```python
from build123d import *
from OCP.BRepAlgoAPI import BRepAlgoAPI_Cut
from OCP.TopTools import TopTools_ListOfShape

# Parameters (mm, degrees)
SKETCH1_R                 = 10
SKETCH1_R_2               = 1.35
BOSS_EXTRUDE1_DEPTH       = 3.175
SKETCH2_W                 = 38.058543228
SKETCH2_H                 = 41.75
SKETCH2_R                 = 1.35
BOSS_EXTRUDE2_DEPTH       = 3.175
SKETCH3_W                 = 38.058543228
SKETCH3_H                 = 41.75
SKETCH3_W_2               = 31.708543228
SKETCH3_H_2               = 35.4
BOSS_EXTRUDE3_DEPTH       = 20
FILLET1_R                 = 5
BOSS_EXTRUDE4_OUTLINE_R   = 1
BOSS_EXTRUDE4_OUTLINE_R_2 = 0.698520241
BOSS_EXTRUDE4_OUTLINE_R_3 = 0.699131638
BOSS_EXTRUDE4_DEPTH       = 4.524579022
SKETCH6_R                 = 0.699665004
SKETCH6_R_2               = 0.703272365
SKETCH6_R_3               = 0.700673295
SKETCH6_R_4               = 0.698053945
BOSS_EXTRUDE5_DEPTH       = 5.225420978
CUT_EXTRUDE3_DEPTH        = 39.629021569
CUT_EXTRUDE4_DEPTH        = 44.672508997
FILLET2_R                 = 1


with BuildPart() as part:
    # Sketch1 → Boss-Extrude1 (new body)
    with BuildSketch(Plane(origin=(0, 0, 0), x_dir=(1, 0, 0), z_dir=(0, 1, 0))):
        with Locations(Location((0, 0, 0), (0, 0, 270))):
            Circle(SKETCH1_R)
        with Locations(Location((0, 7, 0), (0, 0, 270))):
            Circle(SKETCH1_R_2, mode=Mode.SUBTRACT)
        with Locations(Location((7, 0, 0), (0, 0, 270))):
            Circle(SKETCH1_R_2, mode=Mode.SUBTRACT)
        with Locations(Location((0, -7, 0), (0, 0, 270))):
            Circle(SKETCH1_R_2, mode=Mode.SUBTRACT)
        with Locations(Location((-7, 0, 0), (0, 0, 270))):
            Circle(SKETCH1_R_2, mode=Mode.SUBTRACT)
    extrude(amount=BOSS_EXTRUDE1_DEPTH)

    # Sketch2 → Boss-Extrude2 (add)
    with BuildSketch(Plane(origin=(0, 3.175, 0), x_dir=(1, 0, 0), z_dir=(0, 1, 0))):
        Rectangle(SKETCH2_W, SKETCH2_H)
        with Locations(Location((0, -7, 0), (0, 0, 270))):
            Circle(SKETCH2_R, mode=Mode.SUBTRACT)
        with Locations(Location((7, 0, 0), (0, 0, 270))):
            Circle(SKETCH2_R, mode=Mode.SUBTRACT)
        with Locations(Location((-7, 0, 0), (0, 0, 270))):
            Circle(SKETCH2_R, mode=Mode.SUBTRACT)
        with Locations(Location((0, 7, 0), (0, 0, 270))):
            Circle(SKETCH2_R, mode=Mode.SUBTRACT)
    extrude(amount=BOSS_EXTRUDE2_DEPTH)

    # Sketch3 → Boss-Extrude3 (add)
    with BuildSketch(Plane(origin=(0, 6.35, 0), x_dir=(1, 0, 0), z_dir=(0, 1, 0))):
        Rectangle(SKETCH3_W, SKETCH3_H)
        Rectangle(SKETCH3_W_2, SKETCH3_H_2, mode=Mode.SUBTRACT)
    extrude(amount=BOSS_EXTRUDE3_DEPTH)

    # Fillet1
    fillet1_edges = [part.edges().sort_by_distance(p)[0] for p in [
        (-19.029271614, 14.7625, -20.875),
        (-19.029271614, 14.7625, 20.875),
        (19.029271614, 14.7625, 20.875),
        (19.029271614, 14.7625, -20.875),
    ]]
    fillet(fillet1_edges, radius=FILLET1_R)

    # Boss-Extrude4: read off the stored shape, not the designer's step
    # Boss-Extrude4 outline → Boss-Extrude4 (add)
    # profile 1 of 2: a face of its own
    with BuildSketch(Plane.XY.offset(16.350420978)):
        with BuildLine():
            ThreePointArc((9.674791631, 35.998523082), (9.427181956, 35.932908065), (9.244559074, 35.753284112))
            ThreePointArc((9.244559074, 35.753284112), (8.147643376, 34.213929311), (6.807481387, 32.880961337))
            Line((6.807481387, 32.880961337), (6.807482447, 6.35))
            Line((6.807482447, 6.35), (11.963760646, 6.35))
            Line((11.963760646, 6.35), (11.963760646, 35.998520144))
            Line((11.963760646, 35.998520144), (9.674791631, 35.998523082))
        make_face()
        with Locations((9.857482447, 33.16)):
            Circle(BOSS_EXTRUDE4_OUTLINE_R, mode=Mode.SUBTRACT)
        with Locations((9.857482447, 12.46)):
            Circle(BOSS_EXTRUDE4_OUTLINE_R, mode=Mode.SUBTRACT)
    # profile 2 of 2: a face of its own
    with BuildSketch(Plane.XY.offset(16.350420978)):
        with BuildLine():
            Line((-12.751066043, 35.998520144), (-12.751066043, 6.35))
            Line((-12.751066043, 6.35), (-7.592517553, 6.35))
            Line((-7.592517553, 6.35), (-7.592516964, 32.880958857))
            ThreePointArc((-7.592516964, 32.880958857), (-8.932679762, 34.213927416), (-10.029597495, 35.753282149))
            ThreePointArc((-10.029597495, 35.753282149), (-10.212218516, 35.932905514), (-10.459826737, 35.998520144))
            Line((-10.459826737, 35.998520144), (-12.751066043, 35.998520144))
        make_face()
        with Locations((-10.642517553, 33.16)):
            Circle(BOSS_EXTRUDE4_OUTLINE_R_2, mode=Mode.SUBTRACT)
        with Locations((-10.642517553, 12.46)):
            Circle(BOSS_EXTRUDE4_OUTLINE_R_3, mode=Mode.SUBTRACT)
    extrude(amount=BOSS_EXTRUDE4_DEPTH)

    # Sketch6 → Boss-Extrude5 (add)
    with BuildSketch(Plane(origin=(0, 0, -15.649579022), x_dir=(-1, 0, 0), z_dir=(0, 0, -1))):
        with BuildLine():
            Line((10.992517553, 24.135), (10.992517553, 30.51))
            Line((10.992517553, 30.51), (7.192517366, 30.510000072))
            Line((7.192517366, 30.510000072), (6.892517553, 30.510000072))
            Line((6.892517553, 30.510000072), (6.892517553, 32.612557612))
            add(Edge.make_bspline(
                [(6.975743415, 32.783855976), (6.958921233, 32.771091761), (6.928542383, 32.73934935), (6.899316538, 32.679660552), (6.892517469, 32.634957243), (6.892517553, 32.612557612)],
                knots=[1.062e-06, 1.062e-06, 1.062e-06, 1.062e-06, 0.322323684, 0.658094096, 1, 1, 1, 1], degree=3, weights=[1, 1, 1, 1, 1, 1]))
            ThreePointArc((6.975743415, 32.783855976), (8.509170356, 34.198162413), (9.744817778, 35.878887355))
            add(Edge.make_bspline(
                [(9.950114528, 35.998516481), (9.923391157, 35.998516414), (9.869066225, 35.989019468), (9.796326784, 35.947026629), (9.759487209, 35.903468994), (9.744817778, 35.878887355)],
                knots=[0, 0, 0, 0, 0.324047023, 0.652881456, 1, 1, 1, 1], degree=3, weights=[1, 1, 1, 1, 1, 1]))
            Line((9.950114528, 35.998516481), (11.752517552, 35.998516481))
            Line((11.752517552, 35.998516481), (13.252517552, 35.998516481))
            Line((13.252517552, 35.998516481), (13.252517552, 6.318190736))
            Line((13.252517552, 6.318190736), (-12.46748245, 6.318190736))
            Line((-12.46748245, 6.318190736), (-12.46748245, 35.998516481))
            Line((-12.46748245, 35.998516481), (-10.96748245, 35.998516481))
            Line((-10.96748245, 35.998516481), (-9.165078771, 35.998516481))
            add(Edge.make_bspline(
                [(-8.959782959, 35.878887832), (-8.974454973, 35.903473814), (-9.011299786, 35.947034481), (-9.084041461, 35.989022268), (-9.138360889, 35.998516579), (-9.165078771, 35.998516481)],
                knots=[3.25e-07, 3.25e-07, 3.25e-07, 3.25e-07, 0.347182134, 0.676017862, 1, 1, 1, 1], degree=3, weights=[1, 1, 1, 1, 1, 1]))
            ThreePointArc((-8.959782959, 35.878887832), (-7.72413548, 34.198162669), (-6.190708414, 32.783856055))
            add(Edge.make_bspline(
                [(-6.107482447, 32.612555023), (-6.107481996, 32.634920643), (-6.114271613, 32.679614721), (-6.143476784, 32.739319032), (-6.173880837, 32.77108775), (-6.190708414, 32.783856055)],
                knots=[0, 0, 0, 0, 0.341381322, 0.677579946, 1, 1, 1, 1], degree=3, weights=[1, 1, 1, 1, 1, 1]))
            Line((-6.107482447, 32.612555023), (-6.107482447, 30.510000072))
            Line((-6.107482447, 30.510000072), (-6.407482262, 30.510000072))
            Line((-6.407482262, 30.510000072), (-10.207482447, 30.51))
            Line((-10.207482447, 30.51), (-10.207482447, 24.135))
            Line((-10.207482447, 24.135), (-9.049769141, 23.654765682))
            Line((-9.049769141, 23.654765682), (-9.049769141, 12.756914674))
            ThreePointArc((-9.049769141, 12.756914674), (-8.698297278, 11.908386539), (-7.849769141, 11.556914678))
            Line((-7.849769141, 11.556914678), (8.634804248, 11.556914678))
            ThreePointArc((8.634804248, 11.556914678), (9.483332385, 11.908386541), (9.834804247, 12.756914678))
            Line((9.834804247, 12.756914678), (9.834804247, 23.654765682))
            Line((9.834804247, 23.654765682), (10.992517553, 24.135))
        make_face()
        with Locations(Location((-9.857482447, 8.71, 0), (0, 0, 180))):
            Circle(SKETCH6_R, mode=Mode.SUBTRACT)
        with Locations(Location((-9.857482447, 33.16, 0), (0, 0, 180))):
            Circle(SKETCH6_R_2, mode=Mode.SUBTRACT)
        with Locations(Location((10.642517553, 33.16, 0), (0, 0, 180))):
            Circle(SKETCH6_R_3, mode=Mode.SUBTRACT)
        with Locations(Location((10.642517553, 8.71, 0), (0, 0, 180))):
            Circle(SKETCH6_R_4, mode=Mode.SUBTRACT)
    extrude(amount=BOSS_EXTRUDE5_DEPTH)

    # Sketch7 → Cut-Extrude3 (cut, through all)
    with BuildSketch(Plane(origin=(0, 26.35, 0), x_dir=(1, 0, 0), z_dir=(0, 1, 0))):
        Polygon((11.963760646, -16.350420978), (11.963760646, -22.528007323), (30.022930958, -23.761888284), (27.696884363, 28.84716935), (12.46748245, 20.875), (12.46748245, 15.649579022), (12.894365171, -16.350420978), align=None)
        Polygon((-12.751066043, -16.350420978), (-12.751066043, -23.761888284), (-21.517724294, -22.528007323), (-21.901635858, 22.206155736), (-13.252517552, 20.875), (-13.252517552, -16.350420978), align=None)
    extrude(amount=-CUT_EXTRUDE3_DEPTH, mode=Mode.SUBTRACT)


with BuildPart() as cut_extrude4_tool:
    # Sketch9 → Cut-Extrude4 (new, through all)
    with BuildSketch(Plane(origin=(-2e-09, 35.998516482, 0), x_dir=(1.0, 6.10309035182258e-11, 0), z_dir=(-6.10309035182258e-11, 1.0, -1.0368003232160358e-14))):
        Polygon((-12.751066041, -19.525420978), (13.891993445, -19.525420978), (13.555046053, -22.524424576), (-19.185008861, -22.524424576), align=None)
        Polygon((-13.25251755, 18.824579022), (15.127467216, 18.824579022), (13.105782864, 23.749676422), (-20.139693138, 23.131939537), align=None)
    extrude(amount=-CUT_EXTRUDE4_DEPTH)


with BuildPart() as part_1:
    add(part.part)

    # Cut-Extrude4: cut by cut_extrude4_tool, with a tolerance
    cut_extrude4_stock = TopTools_ListOfShape()
    cut_extrude4_stock.Append(part_1.part.wrapped)
    cut_extrude4_tools = TopTools_ListOfShape()
    cut_extrude4_tools.Append(cut_extrude4_tool.part.wrapped)
    cut_extrude4_cut = BRepAlgoAPI_Cut()
    cut_extrude4_cut.SetArguments(cut_extrude4_stock)
    cut_extrude4_cut.SetTools(cut_extrude4_tools)
    cut_extrude4_cut.SetFuzzyValue(0.00001)
    cut_extrude4_cut.Build()
    add(Compound.cast(cut_extrude4_cut.Shape()).solids(), mode=Mode.REPLACE)

    # Fillet2
    fillet2_edges = [part_1.edges().sort_by_distance(p)[0] for p in [
        (12.46748245, 19.58675824, -18.824579022),
        (-13.252517551, 19.58675824, -18.824579022),
        (-12.751066042, 19.58675824, 19.525420978),
        (11.963760646, 19.586758241, 19.525420978),
    ]]
    fillet(fillet2_edges, radius=FILLET2_R)


solid = part_1.part
```
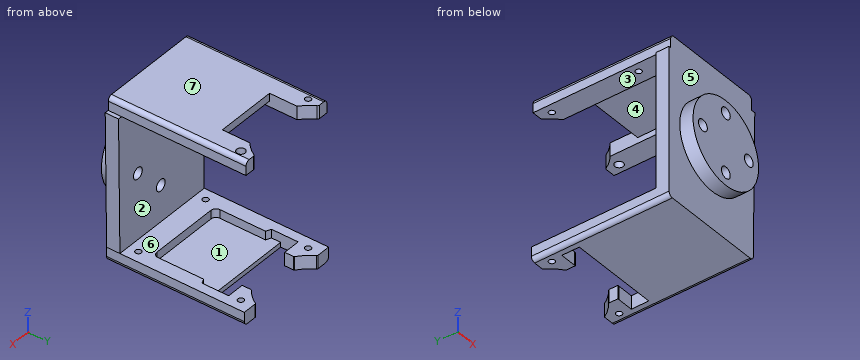
Verification items for the finished model (mm, model axes). Face numbers are marked on the shaded views. A direction names the side the tool comes from. Give positions to 0.01 mm unless a question says otherwise; leave off trailing zeros. Loops run counter-clockwise (first coordinate to the right, second up) from the corner with the lowest first, then second, coordinate; pieces in that order, holes last.
1. Thickness scan on line 1 (Z direction, x = -5.25, y = 24.5); line 2 (Z direction, x = -9, y = 23); line 3 (X direction, y = 16, z = 17.5). Record the ranges inside material, lowest first.
2. Section check A-A, the plane y = 28.5. Enter the section's corners in (x, z), then the cut area to 3 significant figures.
3. Set-up check for the marked faces 4, 5, 6 and 7: record each of +Z, -Z, +X, -X, +Y, -Y from which the full face is reachable in a straight line by a thin tool's end or side.
4. Section check D-D, the plane y = 7.5. Enter the section's corners in (x, z), then the cut area to 3 significant figures.
5. Go/stop test with flat-tipped pins: pin 1 Ø1.5 at (x, z) = (-3.5, 13.5) entering from -Y (3 decimals); pin 2 Ø12 at (x, z) = (-3, -10.5) entering from -Y; pin 3 Ø1 at (y, z) = (27.5, -16.5) entering from +X; pin 4 Ø0.6 at (x, z) = (-4.5, -18) entering from +Y. Record where each tip stops, or that it passes through.
6. Mould release check, pull along Y, two halves, no side actions. Record for the marked faces 1, 2 and 3: released by +Y, released by -Y, zero draft, split by the parting line, or undercut.
7. Section check C-C, the plane x = 0. Enter the section's corners in (y, z) (3 decimals).
8. Section check B-B, the plane z = 7. Enter the section's corners in (x, y) (3 decimals), then the cut area to 3 significant figures.
Geometry says:
1. line 1: z = -18.82 to -17.7, 17.7 to 19.53
1. line 2: z = -18.82 to -17.7, 16.35 to 19.53
1. line 3: x = -12.75 to -7.59, 6.81 to 11.96
2. outline: (-13.25, -17.82) arc R1 ccw to (-12.25, -18.82) - (-10.99, -18.82) - (-10.99, -15.65) - (-13.25, -15.65) - close; (-12.75, 16.35) - (-7.59, 16.35) - (-7.59, 19.53) - (-11.75, 19.53) arc R1 ccw to (-12.75, 18.53) - close; (6.81, 16.35) - (11.96, 16.35) - (11.96, 18.53) arc R1 ccw to (10.96, 19.53) - (6.81, 19.53) - close; (10.21, -18.82) - (11.47, -18.82) arc R1 ccw to (12.47, -17.82) - (12.47, -15.65) - (10.21, -15.65) - close
2. area: 46.2 mm2
3. face 4: +Y
3. face 5: -Y
3. face 6: +X, -X, +Y
3. face 7: +Z, +X, -X, +Y, -Y
4. outline: (-13.25, -17.82) arc R1 ccw to (-12.25, -18.82) - (11.47, -18.82) arc R1 ccw to (12.47, -17.82) - (12.47, -15.65) - (-13.25, -15.65) - close; (-12.75, 16.35) - (-7.59, 16.35) - (-7.59, 17.7) - (6.81, 17.7) - (6.81, 16.35) - (11.96, 16.35) - (11.96, 18.53) arc R1 ccw to (10.96, 19.53) - (-11.75, 19.53) arc R1 ccw to (-12.75, 18.53) - close
4. area: 140 mm2
5. pin 1: stops at y = 3.175
5. pin 2: stops at y = 0
5. pin 3: stops at x = 12.47
5. pin 4: stops at y = 26.35
6. face 1: undercut
6. face 2: released by +Y
6. face 3: zero draft
7. outline: (0, -10) - (3.175, -10) - (3.175, -18.825) - (26.35, -18.825) - (26.35, -17.7) - (11.557, -17.7) - (11.557, -15.65) - (6.35, -15.65) - (6.35, -8.35) - (0, -8.35) - close; (0, -5.65) - (6.35, -5.65) - (6.35, 5.65) - (0, 5.65) - close; (0, 8.35) - (6.35, 8.35) - (6.35, 17.7) - (26.35, 17.7) - (26.35, 19.525) - (3.175, 19.525) - (3.175, 10) - (0, 10) - close
8. outline: (-13.253, 3.175) - (-7.141, 3.175) - (-7.141, 0) - (-1.35, 0) - (-1.35, 6.35) - (-13.253, 6.35) - close; (1.35, 0) - (7.141, 0) - (7.141, 3.175) - (12.77, 3.175) - (12.77, 6.35) - (1.35, 6.35) - close
8. area: 111 mm2
